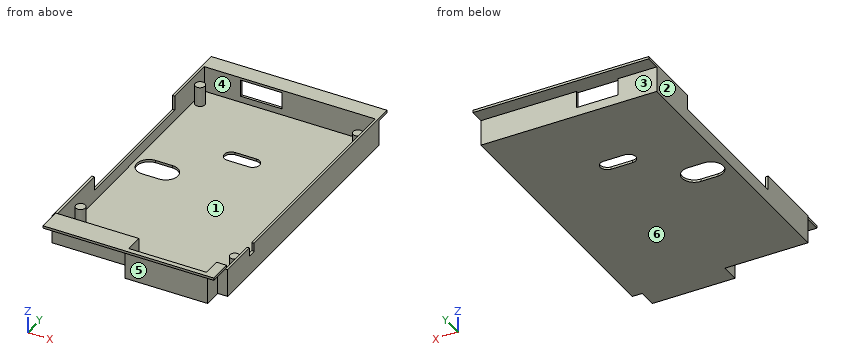
from build123d import *

# Parameters (mm, degrees)
ESBO_O1_W                     = 170.2
ESBO_O1_H                     = 111.2
RESSALTO_EXTRUS_O1_DEPTH      = 0.9
ESBO_O4_W                     = 176.2
ESBO_O4_H                     = 117.2
RESSALTO_EXTRUS_O3_DEPTH      = 1
ESBO_O5_W                     = 32
ESBO_O5_H                     = 1.9
CORTE_EXTRUS_O3_DEPTH         = 5
ESBO_O7_W                     = 70.4
ESBO_O7_H                     = 6
ESBO_O7_H_2                   = 1
RESSALTO_EXTRUS_O4_DEPTH      = 1
ESBO_O7_3_W                   = 70.4
ESBO_O7_3_H                   = 1
RESSALTO_EXTRUS_O5_DEPTH      = 11.6
RESSALTO_EXTRUS_O6_START      = 11.6
RESSALTO_EXTRUS_O6_DEPTH      = 1
RESSALTO_EXTRUS_O7_DEPTH      = 11.6
RESSALTO_EXTRUS_O7_DEPTH_BACK = 1
RESSALTO_EXTRUS_O8_START      = -1
RESSALTO_EXTRUS_O8_DEPTH      = 1
RESSALTO_EXTRUS_O9_DEPTH      = 1
RESSALTO_EXTRUS_O10_DEPTH     = 1
ESBO_O11_W                    = 6
ESBO_O11_H                    = 60
CORTE_EXTRUS_O4_DEPTH         = 1
ESBO_O12_W                    = 3.5
ESBO_O12_H                    = 3.5
CORTE_EXTRUS_O5_DEPTH         = 1
ESBO_O13_W                    = 17
ESBO_O13_H                    = 7
CORTE_EXTRUS_O6_DEPTH         = 1
CORTE_EXTRUS_O7_DEPTH         = 1
CORTE_EXTRUS_O8_DEPTH         = 1
CORTE_EXTRUS_O9_DEPTH         = 215.230343322
CORTE_EXTRUS_O9_DEPTH_BACK    = 215.230343322
ESBO_O17_W                    = 40.80761737
ESBO_O17_H                    = 153.828822039
ESBO_O18_R                    = 2
RESSALTO_EXTRUS_O11_DEPTH     = 8.1


with BuildPart() as part:
    # Esboço1 → Ressalto-extrusão1 (new body)
    with BuildSketch(Plane.XY):
        with Locations((91, 62.6)):
            Rectangle(ESBO_O1_W, ESBO_O1_H)
    extrude(amount=RESSALTO_EXTRUS_O1_DEPTH)

    # Esboço4 → Ressalto-extrusão3 (add)
    with BuildSketch(Plane(origin=(0, 0, 0), x_dir=(-1, 0, 0), z_dir=(0, 0, -1))):
        with Locations((-91, 62.6)):
            Rectangle(ESBO_O4_W, ESBO_O4_H)
    extrude(amount=RESSALTO_EXTRUS_O3_DEPTH)

    # Esboço5 → Corte-extrusão3 (cut)
    with BuildSketch(Plane.XZ.offset(-4)):
        with Locations((91, -0.05)):
            Rectangle(ESBO_O5_W, ESBO_O5_H)
    extrude(amount=-CORTE_EXTRUS_O3_DEPTH, mode=Mode.SUBTRACT)

    # Esboço7 → Ressalto-extrusão4 (add)
    with BuildSketch(Plane(origin=(0, 0, -1), x_dir=(-1, 0, 0), z_dir=(0, 0, -1))):
        with Locations((-75.95, 118.2)):
            Rectangle(ESBO_O7_W, ESBO_O7_H)
        with Locations((-75.95, 114.7)):
            Rectangle(ESBO_O7_W, ESBO_O7_H_2)
    extrude(amount=RESSALTO_EXTRUS_O4_DEPTH)

    # Esboço7<3> → Ressalto-extrusão5 (add)
    with BuildSketch(Plane(origin=(0, 0, -1), x_dir=(-1, 0, 0), z_dir=(0, 0, -1))):
        with Locations((-75.95, 114.7)):
            Rectangle(ESBO_O7_3_W, ESBO_O7_3_H)
    extrude(amount=RESSALTO_EXTRUS_O5_DEPTH)

    # Esboço7<4> → Ressalto-extrusão6 (add)
    with BuildSketch(Plane(origin=(0, 0, -1), x_dir=(-1, 0, 0), z_dir=(0, 0, -1)).offset(RESSALTO_EXTRUS_O6_START)):
        Polygon((-40.75, 114.2), (-111.15, 114.2), (-111.15, 4), (-107, 4), (-107, 9), (-75, 9), (-75, 4), (-40.75, 4), align=None)
        Polygon((-107, 4), (-111.15, 4), (-111.15, 3.5), (-107, 3.5), (-107, -4), (-75, -4), (-75, 3.5), (-40.75, 3.5), (-40.75, 4), (-75, 4), (-75, 9), (-107, 9), align=None)
        Polygon((-107, 3.5), (-111.15, 3.5), (-111.15, 2.5), (-108, 2.5), (-108, -5), (-74, -5), (-74, 2.5), (-40.75, 2.5), (-40.75, 3.5), (-75, 3.5), (-75, -4), (-107, -4), align=None)
    extrude(amount=-RESSALTO_EXTRUS_O6_DEPTH)

    # Esboço7<5> → Ressalto-extrusão7 (add, two sides: drawn at the far end of the back side and taken through both)
    with BuildSketch(Plane(origin=(0, 0, -1), x_dir=(-1, 0, 0), z_dir=(0, 0, -1)).offset(-RESSALTO_EXTRUS_O7_DEPTH_BACK)):
        Polygon((-107, 3.5), (-111.15, 3.5), (-111.15, 2.5), (-108, 2.5), (-108, -5), (-74, -5), (-74, 2.5), (-40.75, 2.5), (-40.75, 3.5), (-75, 3.5), (-75, -4), (-107, -4), align=None)
    extrude(amount=RESSALTO_EXTRUS_O7_DEPTH + RESSALTO_EXTRUS_O7_DEPTH_BACK)

    # Esboço7<6> → Ressalto-extrusão8 (add)
    with BuildSketch(Plane(origin=(0, 0, -1), x_dir=(-1, 0, 0), z_dir=(0, 0, -1)).offset(RESSALTO_EXTRUS_O8_START)):
        Polygon((-74, 2.5), (-40.75, 2.5), (-40.75, -6), (-111.15, -6), (-111.15, 2.5), (-108, 2.5), (-108, -5), (-74, -5), align=None)
    extrude(amount=RESSALTO_EXTRUS_O8_DEPTH)

    # Esboço8 → Ressalto-extrusão9 (add)
    with BuildSketch(Plane(origin=(111.15, 0, 0), x_dir=(0, 0, -1), z_dir=(1, 0, 0))):
        Polygon((1, 121.2), (2, 121.2), (2, 115.2), (12.6, 115.2), (12.6, 2.5), (1, 2.5), align=None)
    extrude(amount=RESSALTO_EXTRUS_O9_DEPTH)

    # Esboço9 → Ressalto-extrusão10 (add)
    with BuildSketch(Plane.ZY.offset(-40.75)):
        Polygon((-2, 121.2), (-1, 121.2), (-1, 2.5), (-12.6, 2.5), (-12.6, 115.2), (-2, 115.2), align=None)
    extrude(amount=RESSALTO_EXTRUS_O10_DEPTH)

    # Esboço11 → Corte-extrusão4 (cut)
    with BuildSketch(Plane.ZY.offset(-39.75)):
        with Locations((-4, 62.2)):
            Rectangle(ESBO_O11_W, ESBO_O11_H)
    extrude(amount=-CORTE_EXTRUS_O4_DEPTH, mode=Mode.SUBTRACT)

    # Esboço12 → Corte-extrusão5 (cut)
    with BuildSketch(Plane(origin=(112.15, 0, 0), x_dir=(0, 0, -1), z_dir=(1, 0, 0))):
        with Locations((2.75, 20.456846579)):
            Rectangle(ESBO_O12_W, ESBO_O12_H)
    extrude(amount=-CORTE_EXTRUS_O5_DEPTH, mode=Mode.SUBTRACT)

    # Esboço13 → Corte-extrusão6 (cut)
    with BuildSketch(Plane(origin=(0, 115.2, 0), x_dir=(1, 0, 0), z_dir=(0, 1, 0))):
        with Locations((64.25, 5.5)):
            Rectangle(ESBO_O13_W, ESBO_O13_H)
    extrude(amount=-CORTE_EXTRUS_O6_DEPTH, mode=Mode.SUBTRACT)

    # Esboço14 → Corte-extrusão7 (cut)
    with BuildSketch(Plane(origin=(0, 0, -12.6), x_dir=(-1, 0, 0), z_dir=(0, 0, -1))):
        with BuildLine():
            Line((-54.178505269, 66.2), (-47.245781338, 66.2))
            ThreePointArc((-47.245781338, 66.2), (-42.245781338, 61.2), (-47.245781338, 56.2))
            Line((-47.245781338, 56.2), (-54.178505269, 56.2))
            ThreePointArc((-54.178505269, 56.2), (-59.178505269, 61.2), (-54.178505269, 66.2))
        make_face()
    extrude(amount=-CORTE_EXTRUS_O7_DEPTH, mode=Mode.SUBTRACT)

    # Esboço15 → Corte-extrusão8 (cut)
    with BuildSketch(Plane(origin=(0, 0, -12.6), x_dir=(-1, 0, 0), z_dir=(0, 0, -1))):
        with BuildLine():
            Line((-78.65004231, 84.60004231), (-69.84995769, 84.60004231))
            ThreePointArc((-69.84995769, 84.60004231), (-66.949915379, 81.7), (-69.84995769, 78.79995769))
            Line((-69.84995769, 78.79995769), (-78.65004231, 78.79995769))
            ThreePointArc((-78.65004231, 78.79995769), (-81.550084621, 81.7), (-78.65004231, 84.60004231))
        make_face()
    extrude(amount=-CORTE_EXTRUS_O8_DEPTH, mode=Mode.SUBTRACT)

    # Esboço17 → Corte-extrusão9 (cut, two sides: drawn at the far end of the back side and taken through both)
    with BuildSketch(Plane(origin=(179.1, 0, 0), x_dir=(0, 0, -1), z_dir=(1, 0, 0)).offset(-CORTE_EXTRUS_O9_DEPTH_BACK)):
        with Locations((-19.403808685, 80.91441102)):
            Rectangle(ESBO_O17_W, ESBO_O17_H)
    extrude(amount=CORTE_EXTRUS_O9_DEPTH + CORTE_EXTRUS_O9_DEPTH_BACK, mode=Mode.SUBTRACT)

    # Esboço18 → Ressalto-extrusão11 (add)
    with BuildSketch(Plane.XY.offset(-11.6)):
        with Locations((43.3, 106.45)):
            Circle(ESBO_O18_R)
        with Locations((108.3, 106.45)):
            Circle(ESBO_O18_R)
        with Locations((108.3, 14.75)):
            Circle(ESBO_O18_R)
        with Locations((44, 16.15)):
            Circle(ESBO_O18_R)
    extrude(amount=RESSALTO_EXTRUS_O11_DEPTH)


solid = part.part
Work out the finished part from the listing and answer in its coordinate system (mm). Face numbers are marked on the shaded views. A direction names the side the tool comes from. Give positions to 0.01 mm unless a question says otherwise; leave off trailing zeros. Order: outer loops, then holes, each group sorted by start corner. A loop starts at its lowest first (then second) coordinate and runs counter-clockwise, first axis right, second up. Notation, with made-up numbers: (71.25, -19) -> (89.25, -19) arc R9 cw to (89.25, -12) -> close; hole circle Ø7 at (-23.5, 47.25). An arc over 180 degrees is marked (long way). One line per item, written item: value.
Item 1: Flat-ended cylindrical pins translate along their axes: P1, Ø4, axis at x = 69, y = 43.5, coming from the +Z side; P2, Ø1, axis at x = 73, z = -8.5, coming from the +Y side; P3, Ø0.8, axis at x = 40.5, y = 69, coming from the +Z side; P4, Ø6, axis at y = 0, z = -4.5, coming from the +X side. Find the tip coordinate at first contact, or state that the pin passes through.
Answer sheet:
P1: z = -11.6
P2: y = 115.2
P3: z = -7
P4: x = 112.15
Item 2: Find section D-D, the plane y = 25.5. Give the vertices of the cut face in (x, z).
Answer sheet:
outline: (39.75, -12.6) -> (112.15, -12.6) -> (112.15, -1) -> (111.15, -1) -> (111.15, -11.6) -> (40.75, -11.6) -> (40.75, -1) -> (39.75, -1) -> close
Item 3: Straight lines are drawn through the part: probe 1 along Y at (x, z) = (97.5, -4); probe 2 along X at (y, z) = (92.5, -3.5); probe 3 along Y at (x, z) = (80, -1.25). For each, find the intervals that lie inside material, in ascending order.
Answer sheet:
probe 1: -5 to -4, 114.2 to 115.2
probe 2: 39.75 to 40.75, 111.15 to 112.15
probe 3: -5 to -4, 114.2 to 121.2
Item 4: Find section C-C, the plane y = 81.7. Give the vertices of the cut face in (x, z), plus the area to 3 significant figures.
Answer sheet:
outline: (39.75, -12.6) -> (66.95, -12.6) -> (66.95, -11.6) -> (40.75, -11.6) -> (40.75, -7) -> (39.75, -7) -> close; (81.55, -12.6) -> (112.15, -12.6) -> (112.15, -1) -> (111.15, -1) -> (111.15, -11.6) -> (81.55, -11.6) -> close
area: 73.0 mm²
Item 5: Find section A-A, the plane y = 61.2. Give the vertices of the cut face in (x, z), plus the area to 3 significant figures.
Answer sheet:
outline: (39.75, -12.6) -> (42.25, -12.6) -> (42.25, -11.6) -> (40.75, -11.6) -> (40.75, -7) -> (39.75, -7) -> close; (59.18, -12.6) -> (112.15, -12.6) -> (112.15, -1) -> (111.15, -1) -> (111.15, -11.6) -> (59.18, -11.6) -> close
area: 70.7 mm²
Item 6: Find section B-B, the plane x = 93.5. Give the vertices of the cut face in (y, z), plus the area to 3 significant figures.
Answer sheet:
outline: (-6, -1) -> (-5, -1) -> (-5, -12.6) -> (115.2, -12.6) -> (115.2, -2) -> (121.2, -2) -> (121.2, -1) -> (114.2, -1) -> (114.2, -11.6) -> (-4, -11.6) -> (-4, 0) -> (-6, 0) -> close
area: 149 mm²
Item 7: Determine the mould class of the marked faces 3, 4, 5 and 6 for opening direction Y: released by +Y, released by -Y, zero draft, split by the parting line, or undercut.
Answer sheet:
face 3: released by +Y
face 4: undercut
face 5: released by -Y
face 6: zero draft
Item 8: A tool of negligible diameter and unlimited length cuts with its end or side. For the marked faces 1 and 2, from which of +Z, -Z, +X, -X, +Y, -Y can it reach the whole face along a straight path? Write none if from no direction.
Answer sheet:
face 1: +Z
face 2: +Z, -Z, -X, +Y, -Y
